from build123d import *

# Parameters (mm, degrees)
SKETCH1_R         = 19
SKETCH1_R_2       = 5.5
EXTRUDE_1_4_DEPTH = 6.35
SKETCH2_R         = 2.75
M5_THROUGH_DEPTH  = 6.35


with BuildPart() as part:
    # Sketch1 → 1/4 (new body)
    with BuildSketch(Plane.XY):
        Circle(SKETCH1_R)
        Circle(SKETCH1_R_2, mode=Mode.SUBTRACT)
    extrude(amount=EXTRUDE_1_4_DEPTH)

    # Sketch2 → M5_through (cut)
    with BuildSketch(Plane.XY):
        with Locations((0, 13.5)):
            Circle(SKETCH2_R)
        with Locations((11.691342951, 6.75)):
            Circle(SKETCH2_R)
        with Locations((11.691342951, -6.75)):
            Circle(SKETCH2_R)
        with Locations((0, -13.5)):
            Circle(SKETCH2_R)
        with Locations((-11.691342951, -6.75)):
            Circle(SKETCH2_R)
        with Locations((-11.691342951, 6.75)):
            Circle(SKETCH2_R)
    extrude(amount=M5_THROUGH_DEPTH, mode=Mode.SUBTRACT)


solid = part.part
Geometry: final body of the model. Coordinates: model frame, mm. Give positions to 0.01 mm unless a question says otherwise; leave off trailing zeros. Loops run counter-clockwise (first coordinate to the right, second up) from the corner with the lowest first, then second, coordinate; pieces in that order, holes last. Notation, with made-up numbers: (-9, 21) -> (28, 21) arc R22 cw to (28, 30) -> close; hole circle Ø2 at (75.25, -31). An arc over 180 degrees is marked (long way). Put each result on its own line as item: value.
1. Cut plane B-B (y = 0). Return the cut outline in (x, z).
Taken from the geometry:
outline: (-19, 0) -> (-5.5, 0) -> (-5.5, 6.35) -> (-19, 6.35) -> close; (5.5, 0) -> (19, 0) -> (19, 6.35) -> (5.5, 6.35) -> close
2. Cut plane C-C (z = 1). Return the cut outline in (x, y), plus the area to 3 significant figures.
Taken from the geometry:
outline: circle Ø38 at (0, 0); hole circle Ø5.5 at (-11.69, -6.75); hole circle Ø5.5 at (-11.69, 6.75); hole circle Ø11 at (0, 0); hole circle Ø5.5 at (0, -13.5); hole circle Ø5.5 at (0, 13.5); hole circle Ø5.5 at (11.69, -6.75); hole circle Ø5.5 at (11.69, 6.75)
area: 897 mm2
3. Ray query, line 1 along Y through (x, z) = (0, 4.5); line 2 along Y through (x, z) = (-10, 4); line 3 along Y through (x, z) = (-1, 4.5). Return the intervals inside material, ascending. Write a range as [from, to].
Taken from the geometry:
line 1: y = [-19, -16.25], [-10.75, -5.5], [5.5, 10.75], [16.25, 19]
line 2: y = [-16.16, -8.92], [-4.58, 4.58], [8.92, 16.16]
line 3: y = [-18.97, -16.06], [-10.94, -5.41], [5.41, 10.94], [16.06, 18.97]
4. Cut plane A-A (x = 0). Return the cut outline in (y, z), plus the area to 3 significant figures.
Taken from the geometry:
outline: (-19, 0) -> (-16.25, 0) -> (-16.25, 6.35) -> (-19, 6.35) -> close; (-10.75, 0) -> (-5.5, 0) -> (-5.5, 6.35) -> (-10.75, 6.35) -> close; (5.5, 0) -> (10.75, 0) -> (10.75, 6.35) -> (5.5, 6.35) -> close; (16.25, 0) -> (19, 0) -> (19, 6.35) -> (16.25, 6.35) -> close
area: 102 mm2
5. Pin query (flat end, axial travel): P1, Ø1.5, axis at x = -10.5, y = -8, coming from the -Z side; P2, Ø1, axis at x = -6.5, z = 3, coming from the +Y side; P3, Ø2, axis at x = 2, z = 0.5, coming from the -Y side; P4, Ø1, axis at x = -4, z = 2.5, coming from the +Y side. Return the tip coordinate at first contact, or that it passes through.
Taken from the geometry:
P1: passes through
P2: stops at y = 18.03
P3: stops at y = -18.97
P4: stops at y = 18.67
6. Cut plane D-D (x = 5). Return the cut outline in (y, z).
Taken from the geometry:
outline: (-18.33, 0) -> (-2.29, 0) -> (-2.29, 6.35) -> (-18.33, 6.35) -> close; (2.29, 0) -> (18.33, 0) -> (18.33, 6.35) -> (2.29, 6.35) -> close
7. Pull-direction query (X, two-part tool) for faces 1 (the cylindrical face through (8.767, -16.856, 3.131)), 2 (the cylindrical face through (-1.19, -5.37, 3.13)), 3 (the flat face through (4, -4, 0)); classes: released by +X, released by -X, zero draft, split by the parting line, or undercut.
Taken from the geometry:
face 1: split by the parting line
face 2: undercut
face 3: zero draft
